Autodesk Inventor part; units mm, degrees
ref_plane "YZ Plane" through (0, 0, 0) normal (1, 0, 0) x (0, 1, 0)
ref_plane "XZ Plane" through (0, 0, 0) normal (0, 1, 0) x (-1, 0, 0)
ref_plane "XY Plane" through (0, 0, 0) normal (0, 0, 1) x (1, 0, 0)
sketch "Sketch6" plane through (0, 0, 0) normal (0, 0, 1) x (1, 0, 0)
  circle A0 centre (0, 0) radius 88.9
  dimension "d25" = 177.8
extrude "Extrusion6" add sketch "Sketch6" along normal blind 368.3
sketch "Sketch7" plane through (0, 0, 368.3) normal (0, 0, 1) x (1, 0, 0)
  circle A0 centre (0, 0) radius 88.9
  line L0 (55.8771, -69.1444) -> (55.8771, -114.3)
  line L1 (-55.8771, -69.1444) -> (-55.8771, -114.3)
  line L2 (-55.8771, -114.3) -> (55.8771, -114.3)
  arc A1 (-55.8771, -69.1444) -> (55.8771, -69.1444) centre (0, 0) ccw
  line L3 (52.7021, -111.125) -> (52.7021, -75.5003)
  arc A2 (-52.7021, -75.5003) -> (52.7021, -75.5003) centre (0, 0) ccw
  line L4 (-52.7021, -75.5003) -> (-52.7021, -111.125)
  line L5 (-52.7021, -111.125) -> (52.7021, -111.125)
  dimension "d29" = 3.175
extrude "Extrusion7" add sketch "Sketch7" against normal blind 368.3 contours A0 L0 L2 L1
fillet "Fillet1" radius 3.175 4 edges at (0, 88.9, 368.3) (0, 88.9, 0) (0, -92.075, 368.3) (0, -92.075, 0)
properties part number "Tank"
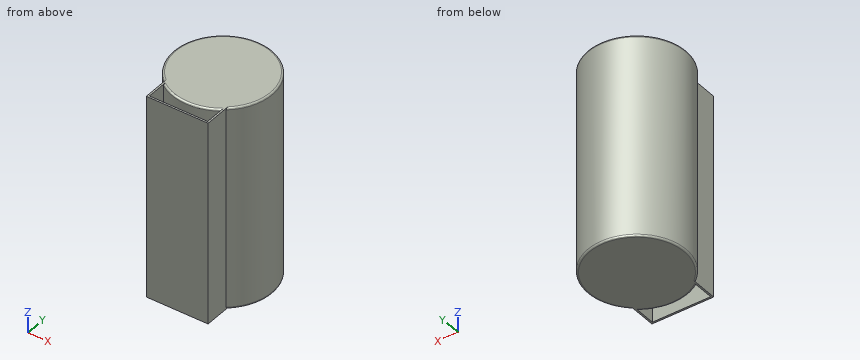
Geometry check sheet. Reference: the model listing, model coordinates, mm. Give positions to 0.01 mm unless a question says otherwise; leave off trailing zeros. Order: outer loops, then holes, each group sorted by start corner. A loop starts at its lowest first (then second) coordinate and runs counter-clockwise, first axis right, second up.
1. Section check A-A, the plane y = -97. Enter the section's corners in (x, z), and give its area (3 significant figures).
2. Section check B-B, the plane x = 0. Enter the section's corners in (y, z) (3 decimals), and give its area (3 significant figures).
3. Thickness scan on L1, parallel to X at y = -103.5, z = 209; L2, parallel to Y at x = -4, z = 275 (3 decimals); L3, parallel to Y at x = -51.5, z = 67 (1 decimal). Record the ranges inside material, lowest first.
4. Section check C-C, the plane z = 249. Enter the section's corners in (x, y) (3 decimals).
5. Gauge pin test, flat ends, axial feed: pin 1 Ø12 at (y, z) = (-100, 230.5) entering from +X; pin 2 Ø6 at (y, z) = (-64, 193) entering from -X; pin 3 Ø5 at (y, z) = (38.5, 161) entering from +X. Record the tip position at first contact, or that the pin passes through.
Values follow:
1. outline: (-55.88, 0) - (-52.7, 0) - (-52.7, 368.3) - (-55.88, 368.3) - close; (52.7, 0) - (55.88, 0) - (55.88, 368.3) - (52.7, 368.3) - close
1. area: 2,340 mm2
2. outline: (-114.3, 0) - (-111.125, 0) - (-111.125, 368.3) - (-114.3, 368.3) - close; (-92.075, 3.175) arc R3.175 ccw to (-88.9, 0) - (85.725, 0) arc R3.175 ccw to (88.9, 3.175) - (88.9, 365.125) arc R3.175 ccw to (85.725, 368.3) - (-88.9, 368.3) arc R3.175 ccw to (-92.075, 365.125) - close
2. area: 67,800 mm2
3. L1: x = -55.88 to -52.7, 52.7 to 55.88
3. L2: y = -114.3 to -111.125, -91.988 to 88.81
3. L3: y = -114.3 to -111.1, -76.3 to 72.5
4. outline: (-55.877, -114.3) - (55.877, -114.3) - (55.877, -69.144) arc R88.9 ccw (long way) to (-55.877, -69.144) - close; hole (-52.702, -111.125) - (52.702, -111.125) - (52.702, -75.5) arc R92.075 cw to (-52.702, -75.5) - close
5. pin 1: stops at x = 55.88
5. pin 2: stops at x = -64.67
5. pin 3: stops at x = 81.28
